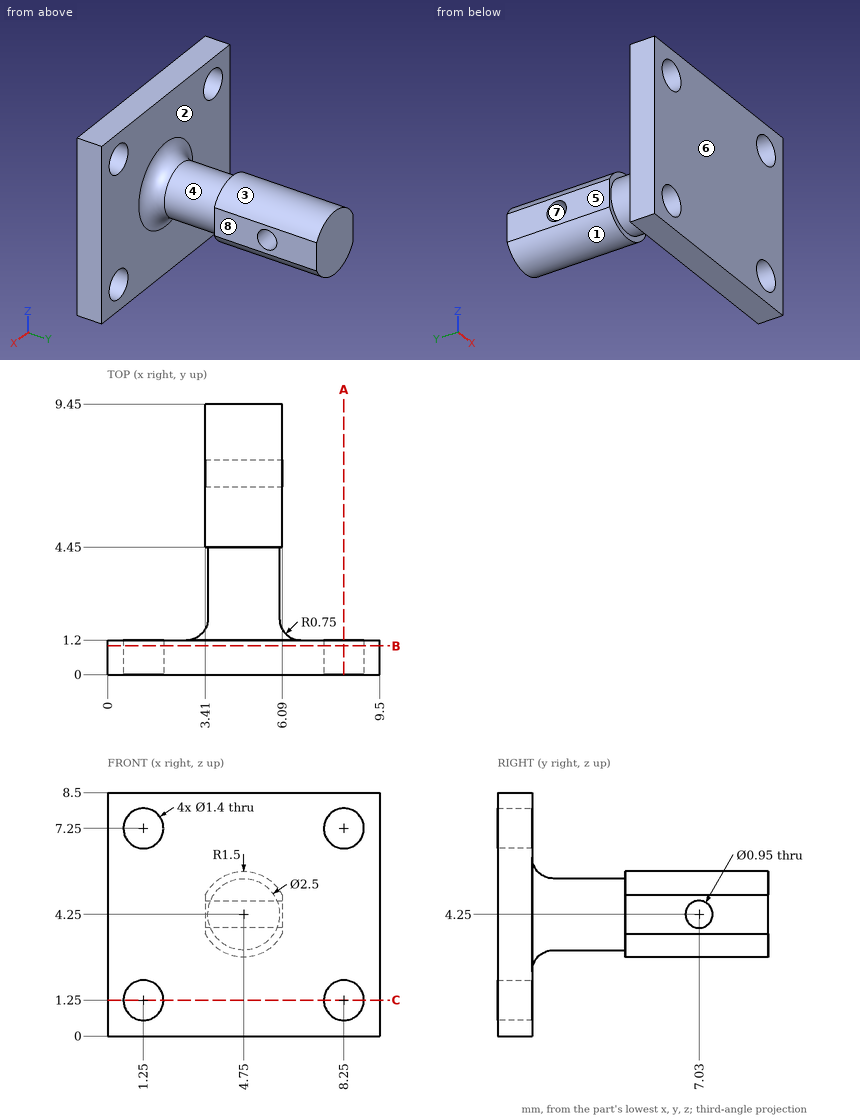
The drawing under review shows one solid part. Ordinate dimensions are in mm from its lowest x, y, z. A direction names the side the tool comes from. Round coordinates to 2 decimals unless told otherwise and drop trailing zeros. Write each loop counter-clockwise with the first axis right and the second up, starting at its lowest first coordinate (ties: lowest second). Pieces come first, ordered by that corner, then holes. Notation, with made-up numbers: (66.5, 41) -> (119.5, 41) arc R13 cw to (119.5, 59) -> close; hole circle Ø9 at (78.25, 22). An arc over 180 degrees is marked (long way). Put each result on its own line as item: value.
Q1. Clearance check with flat-ended pins moving along their axes: pin 1 Ø2 at (x, y) = (6.5, 1.5) entering from -Z; pin 2 Ø1 at (x, y) = (6, 3) entering from +Z; pin 3 Ø3 at (x, y) = (6.5, 3) entering from -Z (1 decimal); pin 4 Ø2 at (x, z) = (1.25, 7.25) entering from +Y. State where each tip first meets the part, or that it passes through.
Determined:
pin 1: stops at z = 0
pin 2: stops at z = 5.25
pin 3: stops at z = 3
pin 4: stops at y = 1.2
Q2. The part is to be moulded in two halves that separate along Y. For the marked faces 6, 7 and 8, say which applies: released by +Y, released by -Y, zero draft, split by the parting line, or undercut.
Determined:
face 6: released by -Y
face 7: undercut
face 8: zero draft
Q3. To check wall thickness, follow L1, parallel to Z at x = 8.25, y = 0.6; L2, parallel to X at y = 0.4, z = 7.25; L3, parallel to Z at x = 1.75, y = 0.75. State the ranges of each line that lie inside material, in increasing order. Write a range as [from, to].
Determined:
L1: z = [0, 0.55], [1.95, 6.55], [7.95, 8.5]
L2: x = [0, 0.55], [1.95, 7.55], [8.95, 9.5]
L3: z = [0, 0.76], [1.74, 6.76], [7.74, 8.5]
Q4. Consider section B-B on y = 1. State the section outline as (x, z) points.
Determined:
outline: (0, 0) -> (9.5, 0) -> (9.5, 8.5) -> (0, 8.5) -> close; hole circle Ø1.4 at (1.25, 1.25); hole circle Ø1.4 at (1.25, 7.25); hole circle Ø1.4 at (8.25, 1.25); hole circle Ø1.4 at (8.25, 7.25)
Q5. Machinability: for the marked faces 1, 2, 3, 4 and 5, which of the approach directions +Z, -Z, +X, -X, +Y, -Y give a long, thin tool a straight path to every point of the face, cutting with its end or side? Answer none if there is none.
Determined:
face 1: -Z, +Y
face 2: +Y
face 3: +Z, +Y
face 4: none
face 5: +Z, -Z, -X, +Y
Q6. Consider section C-C on z = 1.25. State the section outline as (x, y) points.
Determined:
outline: (0, 0) -> (0.55, 0) -> (0.55, 1.2) -> (0, 1.2) -> close; (1.95, 0) -> (7.55, 0) -> (7.55, 1.2) -> (1.95, 1.2) -> close; (8.95, 0) -> (9.5, 0) -> (9.5, 1.2) -> (8.95, 1.2) -> close
Q7. Consider section A-A on x = 8.25. State the section outline as (y, z) points.
Determined:
outline: (0, 0) -> (1.2, 0) -> (1.2, 0.55) -> (0, 0.55) -> close; (0, 1.95) -> (1.2, 1.95) -> (1.2, 6.55) -> (0, 6.55) -> close; (0, 7.95) -> (1.2, 7.95) -> (1.2, 8.5) -> (0, 8.5) -> close
